Verification items for the finished model (mm, model axes). Face numbers are marked on the shaded views. Give positions to 0.01 mm unless a question says otherwise; leave off trailing zeros. Loops run counter-clockwise (first coordinate to the right, second up) from the corner with the lowest first, then second, coordinate; pieces in that order, holes last. Notation, with made-up numbers: M -34.5,55.25 L -6.5,55.25 A18 cw -6.5,79.25 Z; hole C 19,44 d10. An arc over 180 degrees is marked long. Use CSV: the item, a comma, the result in double quotes.
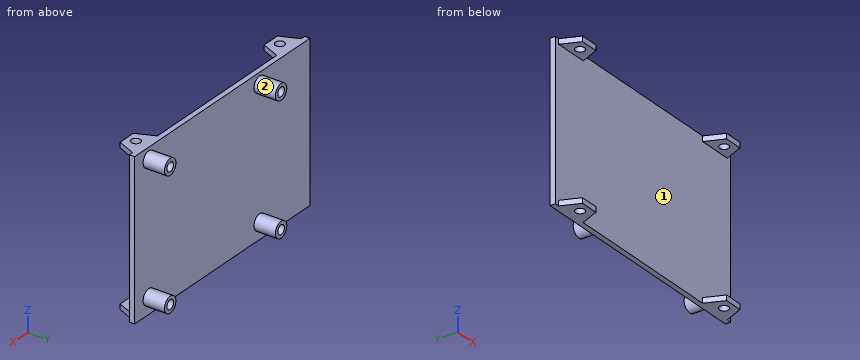
Autodesk Inventor part; units mm, degrees
ref_plane "YZ Plane" through (0, 0, 0) normal (1, 0, 0) x (0, 1, 0)
ref_plane "XZ Plane" through (0, 0, 0) normal (0, 1, 0) x (-1, 0, 0)
ref_plane "XY Plane" through (0, 0, 0) normal (0, 0, 1) x (1, 0, 0)
sketch "Sketch1" plane through (0, 0, 0) normal (0, 1, 0) x (-1, 0, 0)
  line L0 (0, 0) -> (92.5, 0)
  line L1 (92.5, 0) -> (92.5, -59.5)
  line L2 (92.5, -59.5) -> (0, -59.5)
  line L3 (0, -59.5) -> (0, 0)
  dimension "d0" = 92.5
  dimension "d1" = 59.5
extrude "Extrusion1" add sketch "Sketch1" along normal blind 2
sketch "Sketch2" plane through (0, 0, -59.5) normal (0, 0, -1) x (-1, 0, 0)
  line L0 (0, 0) -> (92.5, 0)
  line L1 (46.25, 0) -> (46.25, 2) construction
  line L2 (92.5, 2) -> (0, 2)
  line L3 (14.75, 0) -> (1.75, 0)
  line L4 (4.75, -7) -> (11.75, -7)
  line L5 (1.75, 0) -> (4.75, -7)
  line L6 (14.75, 0) -> (11.75, -7)
  circle A0 centre (8.25, -3.5) radius 1.75
  line L7 (87.75, -7) -> (80.75, -7)
  line L8 (90.75, 0) -> (87.75, -7)
  line L9 (77.75, 0) -> (80.75, -7)
  circle A1 centre (84.25, -3.5) radius 1.75
  line L10 (90.75, 0) -> (77.75, 0)
  dimension "d4" = 13
  dimension "d5" = 7
  dimension "d6" = 1.75
  dimension "d7" = 7
  dimension "d8" = 3
  dimension "d9" = 3.5
  dimension "d10" = 6.5
  dimension "d11" = 3.5
extrude "Extrusion2" add sketch "Sketch2" against normal up to surface (59.5 mm away)
sketch "Sketch3" plane through (0, 0, 0) normal (0, -1, 0) x (1, 0, 0)
  line L0 (-92.5, -57.5) -> (0, -57.5)
  line L1 (0, -57.5) -> (0, -2)
  line L2 (0, -2) -> (-92.5, -2)
  line L3 (-92.5, -2) -> (-92.5, -57.5)
  line L4 (-77.75, -59.5) -> (-14.75, -59.5)
  line L5 (-92.5, -59.5) -> (-92.5, 0)
  line L6 (-14.75, 0) -> (-77.75, 0)
  line L7 (0, 0) -> (0, -59.5)
  dimension "d14" = 2
  dimension "d16" = 0
  dimension "d17" = 2
  dimension "d18" = 0
extrude "Extrusion3" cut sketch "Sketch3" along normal through all
sketch "Sketch4" plane through (0, 2, 0) normal (0, 1, 0) x (1, 0, 0)
  line L0 (-89, 0.8) -> (-4, 0.8) construction
  line L1 (-4, 0.8) -> (-4, 56.8) construction
  line L2 (-4, 56.8) -> (-89, 56.8) construction
  line L3 (-89, 56.8) -> (-89, 0.8) construction
  line L4 (0, 0) -> (0, 59.5)
  line L5 (-92.5, 0) -> (0, 0)
  circle A0 centre (-7.5, 4.3) radius 3
  circle A1 centre (-7.5, 53.3) radius 3
  circle A2 centre (-66, 4.3) radius 3
  circle A3 centre (-66, 53.3) radius 3
  circle A4 centre (-66, 4.3) radius 1.75
  circle A5 centre (-66, 53.3) radius 1.75
  circle A6 centre (-7.5, 53.3) radius 1.75
  circle A7 centre (-7.5, 4.3) radius 1.75
  dimension "d21" = 85
  dimension "d22" = 56
  dimension "d23" = 4
  dimension "d24" = 0.8
  dimension "d25" = 6
  dimension "d26" = 6
  dimension "d27" = 6
  dimension "d28" = 6
  dimension "d29" = 3.5
  dimension "d30" = 3.5
  dimension "d31" = 3.5
  dimension "d32" = 3.5
  dimension "d33" = 3.5
  dimension "d34" = 3.5
  dimension "d35" = 58.5
  dimension "d36" = 58.5
  dimension "d37" = 3.5
  dimension "d38" = 3.5
  dimension "d39" = 3.5
  dimension "d40" = 3.5
extrude "Extrusion4" add sketch "Sketch4" along normal blind 8.2
properties part number "Pi Holder"
(1) Depth check by flat-ended pin: pin 1 Ø4 at (x, z) = (-7.5, -4.3) entering from -Y; pin 2 Ø3 at (x, z) = (-66, -4.5) entering from +Y. Enter the tip coordinate at first touch or a pass-through.
Calculated:
pin 1,"stops at y = 0"
pin 2,"stops at y = 2"
(2) Scan lines: L1, parallel to Z at x = -66, y = 5; L2, parallel to X at y = 8, z = -53.3; L3, parallel to Z at x = -6, y = -4. Record each from-to range of solid material in increasing order. Write a range as from..to.
Calculated:
L1,"z = -56.3..-55.05, -51.55..-50.3, -7.3..-6.05, -2.55..-1.3"
L2,"x = -69..-67.75, -64.25..-63, -10.5..-9.25, -5.75..-4.5"
L3,"z = -59.5..-57.5, -2..0"
(3) Section check A-A on y = 3.25. Record the cut outline in (x, z), plus the area to 3 significant figures.
Calculated:
outline,"C -66,-53.3 d6; C -66,-4.3 d6; C -7.5,-53.3 d6; C -7.5,-4.3 d6; hole C -66,-53.3 d3.5; hole C -66,-4.3 d3.5; hole C -7.5,-53.3 d3.5; hole C -7.5,-4.3 d3.5"
area,"74.6 mm²"
(4) Section check D-D on x = -7.5. Count the separate pieces of the cut face and the enclosed holes in it, plus the area to 3 significant figures.
Calculated:
separate pieces,"3"
enclosed holes,"0"
area,"175 mm²"
(5) Section check B-B on x = -66. Record the cut outline in (y, z), plus the area to 3 significant figures.
Calculated:
outline,"M 0,-59.5 L 2,-59.5 L 2,-56.3 L 10.2,-56.3 L 10.2,-55.05 L 2,-55.05 L 2,-51.55 L 10.2,-51.55 L 10.2,-50.3 L 2,-50.3 L 2,-7.3 L 10.2,-7.3 L 10.2,-6.05 L 2,-6.05 L 2,-2.55 L 10.2,-2.55 L 10.2,-1.3 L 2,-1.3 L 2,0 L 0,0 Z"
area,"160 mm²"
(6) Section check C-C on z = -4.3. Record the cut outline in (x, y), plus the area to 3 significant figures.
Calculated:
outline,"M -92.5,0 L 0,0 L 0,2 L -4.5,2 L -4.5,10.2 L -5.75,10.2 L -5.75,2 L -9.25,2 L -9.25,10.2 L -10.5,10.2 L -10.5,2 L -63,2 L -63,10.2 L -64.25,10.2 L -64.25,2 L -67.75,2 L -67.75,10.2 L -69,10.2 L -69,2 L -92.5,2 Z"
area,"226 mm²"
(7) Mould release check, pull along Z, two halves, no side actions. Record for the marked faces 1 and 2: released by +Z, released by -Z, zero draft, split by the parting line, or undercut.
Calculated:
face 1,"undercut"
face 2,"undercut"
